Part model, mm, in its own coordinate system. Give positions to 0.01 mm unless a question says otherwise; leave off trailing zeros. Order: outer loops, then holes, each group sorted by start corner. A loop starts at its lowest first (then second) coordinate and runs counter-clockwise, first axis right, second up. Notation, with made-up numbers: M 62.5,-13.75 L 121.5,-13.75 A26 ccw 121.5,8.25 Z; hole C -4,67 d2. An arc over 180 degrees is marked long. Answer as a JSON object with one key per item and string values.
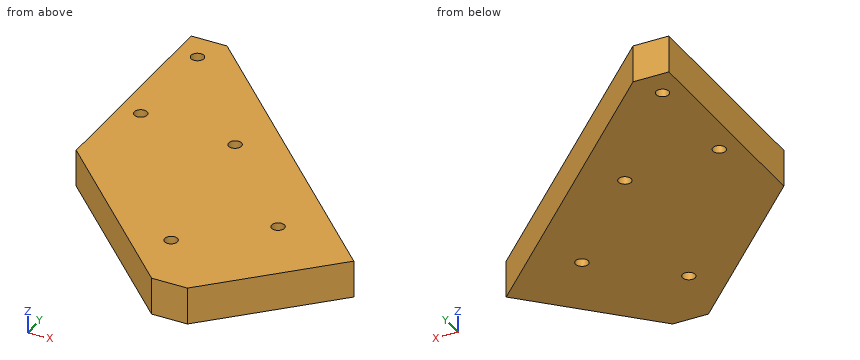
from build123d import *

# Parameters (mm, degrees)
BOSS_EXTRUDE1_DEPTH       = 6.604
F_4_40_TAPPED_HOLE1_D     = 2.2606
F_4_40_TAPPED_HOLE1_DEPTH = 7.5946
F_4_40_TAPPED_HOLE1_TIP   = 0.679152758
CUT_EXTRUDE1_DEPTH        = 7.604


with BuildPart() as part:
    # Sketch1 → Boss-Extrude1 (new body)
    with BuildSketch(Plane.XY):
        Polygon((6.35, -6.35), (53.881536726, -53.881536726), (31.430896424, -76.332177029), (0, -44.901280605), (0, -6.35), align=None)
    extrude(amount=BOSS_EXTRUDE1_DEPTH)

    # #4-40 Tapped Hole1
    with Locations(Plane.XY.offset(6.604)):
        with Locations((3.81, -11.43), (3.81, -30.48), (25.663262225, -61.689692887), (21.210222222, -31.794452992), (38.593017634, -50.314669612)):
            Hole(F_4_40_TAPPED_HOLE1_D / 2, depth=F_4_40_TAPPED_HOLE1_DEPTH)
            with Locations((0, 0, -(F_4_40_TAPPED_HOLE1_DEPTH + F_4_40_TAPPED_HOLE1_TIP / 2))):  # 118° drill point
                Cone(0, F_4_40_TAPPED_HOLE1_D / 2, F_4_40_TAPPED_HOLE1_TIP, mode=Mode.SUBTRACT)

    # Sketch5 → Cut-Extrude1 (cut, through all)
    with BuildSketch(Plane.XY.offset(6.604)):
        Polygon((34.605896424, -73.157177029), (28.255896424, -73.157177029), (31.430896424, -76.332177029), align=None)
    extrude(amount=-CUT_EXTRUDE1_DEPTH, mode=Mode.SUBTRACT)


solid = part.part
1. Cut at D-D on y = -43.5. Give the cut face in (x, z), plus the area to 3 significant figures.
Worked answers:
{"outline": "M 0,0 L 43.5,0 L 43.5,6.6 L 0,6.6 Z", "area": "287 mm^2"}
2. Pin check, flat tips, straight feed: P1, Ø1, axis at x = 18, z = 5.5, coming from the -Y side; P2, Ø2, axis at x = 35, z = 5.5, coming from the +Y side. Stop position of each tip, or through.
Worked answers:
{"P1": "stops at y = -63.4", "P2": "stops at y = -34"}
3. Cut at B-B on x = 3.81. Give the cut face in (y, z).
Worked answers:
{"outline": "M -48.71,0 L -31.61,0 L -31.61,6.6 L -48.71,6.6 Z; M -29.35,0 L -12.56,0 L -12.56,6.6 L -29.35,6.6 Z; M -10.3,0 L -6.35,0 L -6.35,6.6 L -10.3,6.6 Z"}
4. Cut at C-C on z = 0.75. Give the cut face in (x, y).
Worked answers:
{"outline": "M 0,-44.9 L 28.26,-73.16 L 34.61,-73.16 L 53.88,-53.88 L 6.35,-6.35 L 0,-6.35 Z; hole C 3.81,-30.48 d2.26; hole C 3.81,-11.43 d2.26; hole C 21.21,-31.79 d2.26; hole C 25.66,-61.69 d2.26; hole C 38.59,-50.31 d2.26"}
5. Cut at A-A on y = -11.43. Give the cut face in (x, z).
Worked answers:
{"outline": "M 0,0 L 2.68,0 L 2.68,6.6 L 0,6.6 Z; M 4.94,0 L 11.43,0 L 11.43,6.6 L 4.94,6.6 Z"}
6. Probe line 1 along Y through (x, z) = (21.5, 1.75); line 2 along Y through (x, z) = (3.81, 1.5); line 3 along Y through (x, z) = (4, 3). List the from-to ranges inside material, lowest first.
Worked answers:
{"line 1": "y = -66.4 to -32.89, -30.7 to -21.5", "line 2": "y = -48.71 to -31.61, -29.35 to -12.56, -10.3 to -6.35", "line 3": "y = -48.9 to -31.59, -29.37 to -12.54, -10.32 to -6.35"}
